from build123d import *

# Parameters (mm, degrees)
SKETCH1_W           = 21.3
SKETCH1_H           = 15.1
BOSS_EXTRUDE1_DEPTH = 25
BOSS_EXTRUDE2_REACH = 34.289
SKETCH4_W           = 13.6
SKETCH4_H           = 17.676442621


with BuildPart() as part:
    # Sketch1 → Boss-Extrude1 (new body)
    with BuildSketch(Plane(origin=(0, 0, 0), x_dir=(1, 0, 0), z_dir=(0, 1, 0))):
        Rectangle(SKETCH1_W, SKETCH1_H)
    extrude(amount=BOSS_EXTRUDE1_DEPTH)

    # Boss-Extrude2: up to this plane
    boss_extrude2_end = Plane(origin=(0, 25, 0), z_dir=(0, 1, 0))
    # Sketch4 → Boss-Extrude2 (add, up to the surface)
    with BuildSketch(Plane(origin=(-6.963414725, 25.987817547, 0), x_dir=(0, 0, 1), z_dir=(-0.25881904510252474, 0.9659258262890673, 0)), mode=Mode.PRIVATE) as boss_extrude2_sk1:
        with Locations((0, 6.470476128)):
            Rectangle(SKETCH4_W, SKETCH4_H)
    boss_extrude2_tool1 = split(extrude(boss_extrude2_sk1.sketch, amount=-BOSS_EXTRUDE2_REACH, mode=Mode.PRIVATE), bisect_by=boss_extrude2_end, keep=Keep.BOTH, mode=Mode.PRIVATE)
    add(boss_extrude2_tool1.solids().sort_by_distance((-0.713415, 27.6625, 0))[0])


solid = part.part
CAD build for the part. Positions are in the model's coordinates, mm. A direction names the side the tool comes from. Round coordinates to 2 decimals unless told otherwise and drop trailing zeros. Write each loop counter-clockwise with the first axis right and the second up, starting at its lowest first coordinate (ties: lowest second). Pieces come first, ordered by that corner, then holes.
(1) 3-axis set-ups, long thin cutter, end or side, ignore diameter. For faces 4 (the face through (2, 26, -6.8)), 5 (the face through (-10.65, 12, 0)): which of +Z, -Z, +X, -X, +Y, -Y reach the whole face in a straight line?
(2) Slice it at A-A, the plane z = -6.25. Write the cut outline in (x, y) (3 decimals), and give its area (3 significant figures).
(3) Slice it at C-C, the plane y = 26.5. Write the cut outline in (x, z).
(4) Drop flat-ended pins along their axis: P1, Ø6, axis at x = -8, z = 3.5, coming from the -Y side; P2, Ø1.5, axis at x = 4, y = 28.5, coming from the +Z side; P3, Ø6, axis at x = 3.5, z = -1.5, coming from the +Y side. Give the stop position or say it passes through.
(5) Slice it at B-B, the plane x = -4. Write the cut outline in (y, z), and give its area (3 significant figures).
(6) Probe line 1 along Z through (x, y) = (-8.5, 25.5); line 2 along Y through (x, z) = (0.25, -3.5); line 3 along Y through (x, z) = (-9.5, -1.5). List the from-to ranges inside material, lowest first.
(7) Mould opens along Z. For faces 1 (the face through (2, 26, 6.8)), 2 (the face through (0, 0, 0)), 3 (the face through (0, 12, -7.55)) say: pulls with the +Z half, pulls with the -Z half, needs draft (parallel to the pull), parting line crosses it, or undercut.
From the geometry:
1. face 4: -Z, +X, -X, +Y
1. face 5: +Z, -Z, -X, +Y, -Y
2. outline: (-10.65, 0) - (10.65, 0) - (10.65, 25) - (9.15, 25) - (7.824, 29.95) - (-9.25, 25.375) - (-9.15, 25) - (-10.65, 25) - close
2. area: 581 mm2
3. outline: (-5.05, -6.8) - (8.75, -6.8) - (8.75, 6.8) - (-5.05, 6.8) - close
4. P1: stops at y = 0
4. P2: stops at z = 6.8
4. P3: stops at y = 29.6
5. outline: (0, -7.55) - (25, -7.55) - (25, -6.8) - (26.78, -6.8) - (26.78, 6.8) - (25, 6.8) - (25, 7.55) - (0, 7.55) - close
5. area: 402 mm2
6. line 1: z = -6.8 to 6.8
6. line 2: y = 0 to 27.92
6. line 3: y = 0 to 25
7. face 1: pulls with the +Z half
7. face 2: needs draft
7. face 3: pulls with the -Z half
